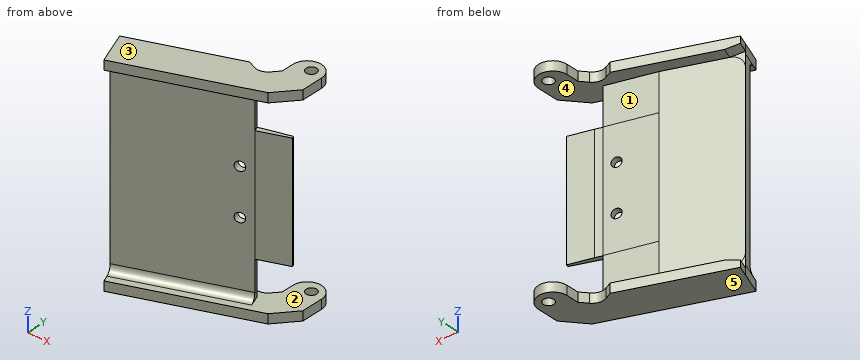
from build123d import *
from OCP.BRepFilletAPI import BRepFilletAPI_MakeChamfer

# Parameters (mm, degrees)
ESTRUSIONE_ESTRUSIONE1_DEPTH = 4
ESTRUSIONE_ESTRUSIONE2_DEPTH = 82
ESTRUSIONE_ESTRUSIONE3_START = 4
ESTRUSIONE_ESTRUSIONE3_DEPTH = 4
FORO_PER_VITE_M4_1_D         = 4.5
FORO_PER_VITE_M4_1_DEPTH     = 188
FORO_PER_VITE_M4_1_TIP       = 1.351936393
SCHIZZO6_W                   = 50
SCHIZZO6_H                   = 4
ESTRUSIONE_ESTRUSIONE4_DEPTH = 5
SMUSSO1_SIZE                 = 5.5
SMUSSO1_SIZE2                = 1.169061089
RACCORDO1_R                  = 3
SMUSSO2_SIZE                 = 5
RACCORDO2_START              = -86
RACCORDO2_DEPTH              = 4
RACCORDO2_2_DEPTH            = 4
SCHIZZO7_W                   = 50
SCHIZZO7_H                   = 2.5
ESTRUSIONE_ESTRUSIONE5_DEPTH = 13
SMUSSO3_SIZE                 = 20
SMUSSO3_SIZE_2               = 1.048155586
SMUSSO4_SIZE                 = 20
SMUSSO4_SIZE2                = 1.749773271
SMUSSO5_SIZE                 = 10
SMUSSO5_SIZE2                = 0.350328071
SCHIZZO8_R                   = 2
TAGLIO_ESTRUSIONE1_DEPTH     = 10


with BuildPart() as part:
    # Schizzo1 → Estrusione-Estrusione1 (new body)
    with BuildSketch(Plane.XY):
        with BuildLine():
            Line((4.891723927, 5.829729564), (4.891723927, 11.038087105))
            ThreePointArc((4.891723927, 11.038087105), (11.08058435, 17.226947528), (17.269444773, 11.038087105))
            Line((17.269444773, 11.038087105), (17.269444773, 1.912236928))
            Line((17.269444773, 1.912236928), (9.899185428, -6.871296125))
            Line((9.899185428, -6.871296125), (-42.94312967, -27.493410377))
            Line((-42.94312967, -27.493410377), (-46.57866514, -18.177677349))
            Line((-46.57866514, -18.177677349), (0, 0))
            Line((0, 0), (4.891723927, 5.829729564))
        make_face()
    extrude(amount=ESTRUSIONE_ESTRUSIONE1_DEPTH)

    # Schizzo4 → Estrusione-Estrusione2 (add)
    with BuildSketch(Plane.XY):
        Polygon((-45.124450952, -21.90397056), (1.454214188, -3.726293211), (0, 0), (-46.57866514, -18.177677349), align=None)
    extrude(amount=-ESTRUSIONE_ESTRUSIONE2_DEPTH)

    # Schizzo5 → Estrusione-Estrusione3 (add)
    with BuildSketch(Plane(origin=(0, 0, -82), x_dir=(-1, 0, 0), z_dir=(0, 0, -1)).offset(ESTRUSIONE_ESTRUSIONE3_START)):
        with BuildLine():
            Line((42.94312967, -27.493410377), (46.57866514, -18.177677349))
            Line((46.57866514, -18.177677349), (0, 0))
            Line((0, 0), (-4.891723927, 5.829729564))
            Line((-4.891723927, 5.829729564), (-4.891723927, 11.038087105))
            ThreePointArc((-4.891723927, 11.038087105), (-11.08058435, 17.226947528), (-17.269444773, 11.038087105))
            Line((-17.269444773, 11.038087105), (-17.269444773, 1.912236928))
            Line((-17.269444773, 1.912236928), (-9.899185428, -6.871296125))
            Line((-9.899185428, -6.871296125), (42.94312967, -27.493410377))
        make_face()
    extrude(amount=-ESTRUSIONE_ESTRUSIONE3_DEPTH)

    # Foro per Vite M4-1
    with Locations(Plane.XY.offset(4)):
        with Locations((11.891723927, 12.226947528)):
            Hole(FORO_PER_VITE_M4_1_D / 2, depth=FORO_PER_VITE_M4_1_DEPTH)
            with Locations((0, 0, -(FORO_PER_VITE_M4_1_DEPTH + FORO_PER_VITE_M4_1_TIP / 2))):  # 118° drill point
                Cone(0, FORO_PER_VITE_M4_1_D / 2, FORO_PER_VITE_M4_1_TIP, mode=Mode.SUBTRACT)

    # Schizzo6 → Estrusione-Estrusione4 (add)
    with BuildSketch(Plane(origin=(0, 0, 0), x_dir=(0.9315733027957475, 0.36355354697516373, 0), z_dir=(-0.36355354697516373, 0.9315733027957475, 0))):
        with Locations((-25, 84)):
            Rectangle(SCHIZZO6_W, SCHIZZO6_H)
        with Locations((-25, -2)):
            Rectangle(SCHIZZO6_W, SCHIZZO6_H)
    extrude(amount=ESTRUSIONE_ESTRUSIONE4_DEPTH)

    # Smusso1: one chamfer whose edges measure the first distance from different faces: ONE call of the kernel's chamfer builder (chamfer() names one face for all edges)
    smusso1_edges_1 = [part.edges().sort_by_distance(p)[0] for p in [
        (-47.487549007, -15.848744092, -82),
    ]]
    smusso1_side_1 = [part.faces().sort_by_distance(p)[0] for p in [
        (-24.198216437, -6.759905417, -82),
    ]]
    smusso1_edges_2 = [part.edges().sort_by_distance(p)[0] for p in [
        (-47.487549007, -15.848744092, 0),
    ]]
    smusso1_side_2 = [part.faces().sort_by_distance(p)[0] for p in [
        (-24.198216437, -6.759905417, 0),
    ]]
    smusso1 = BRepFilletAPI_MakeChamfer(part.part.solid().wrapped)
    for e in smusso1_edges_1:
        smusso1.Add(SMUSSO1_SIZE, SMUSSO1_SIZE2, e.wrapped, smusso1_side_1[0].wrapped)  # the first distance lies on this face
    for e in smusso1_edges_2:
        smusso1.Add(SMUSSO1_SIZE, SMUSSO1_SIZE2, e.wrapped, smusso1_side_2[0].wrapped)  # the first distance lies on this face
    add(Compound.cast(smusso1.Shape()), mode=Mode.REPLACE)

    # Raccordo1
    raccordo1_edges = [part.edges().sort_by_distance(p)[0] for p in [
        (-21.835118382, -12.815131886, -82),
        (-21.835118382, -12.815131886, 0),
    ]]
    fillet(raccordo1_edges, radius=RACCORDO1_R)

    # Smusso2
    smusso2_edges = [part.edges().sort_by_distance(p)[0] for p in [
        (-1.817767735, 4.657866514, 2),
        (-1.817767735, 4.657866514, -84),
    ]]
    chamfer(smusso2_edges, length=SMUSSO2_SIZE - 0.0001)  # a hair under: the kernel refuses the full size

    # Raccordo2: read off the stored shape, not the designer's step
    # Raccordo2 outline → Raccordo2 (add)
    with BuildSketch(Plane.XY.offset(RACCORDO2_START)):
        with BuildLine():
            Line((0, 0), (2.407895765, 2.869618428))
            ThreePointArc((2.407895765, 2.869618428), (-0.284030607, 1.214852073), (-3.430579557, 1.504591587))
            Line((-3.430579557, 1.504591587), (0, 0))
        make_face()
    extrude(amount=RACCORDO2_DEPTH)

    # Raccordo2 2 outline → Raccordo2 2 (add)
    with BuildSketch(Plane.XY):
        with BuildLine():
            Line((0, 0), (2.407895765, 2.869618428))
            ThreePointArc((2.407895765, 2.869618428), (-0.284030607, 1.214852073), (-3.430579557, 1.504591587))
            Line((-3.430579557, 1.504591587), (0, 0))
        make_face()
    extrude(amount=RACCORDO2_2_DEPTH)

    # Schizzo7 → Estrusione-Estrusione5 (add)
    with BuildSketch(Plane(origin=(0, 0, 0), x_dir=(0, 0, -1), z_dir=(0.9315733027957472, 0.3635535469751644, 0))):
        with Locations((41, -2.75)):
            Rectangle(SCHIZZO7_W, SCHIZZO7_H)
    extrude(amount=ESTRUSIONE_ESTRUSIONE5_DEPTH)

    # Smusso3
    # the kernel refuses this chamfer: 20, 1.048155586 mm, written as the material it takes off along each edge
    with BuildSketch(Plane(origin=(12.655783257, 3.328836156, -16), x_dir=(-0.9315733027957472, -0.3635535469751644, 0), z_dir=(0, 0, -1))) as smusso3_piece_1_section:
        Polygon((SMUSSO3_SIZE, 0), (0, -SMUSSO3_SIZE_2), (0, 0), align=None)
    smusso3_piece_1 = extrude(amount=50, mode=Mode.PRIVATE)
    smusso3_piece_1 = split(smusso3_piece_1, bisect_by=Plane(origin=(0.54533032, -1.397359954, -16), z_dir=(0.9315733027957472, 0.36355354697516445, 0)), keep=Keep.TOP, mode=Mode.PRIVATE)
    add(smusso3_piece_1, mode=Mode.SUBTRACT)

    # Smusso4
    smusso4_edges = [part.edges().sort_by_distance(p)[0] for p in [
        (0, 0, -41),
    ]]
    smusso4_side = [part.faces().sort_by_distance(p)[0] for p in [
        (-23.323124739, -9.102026325, -41),
    ]]
    chamfer(smusso4_edges, length=SMUSSO4_SIZE, length2=SMUSSO4_SIZE2, reference=smusso4_side[0])

    # Smusso5
    smusso5_edges = [part.edges().sort_by_distance(p)[0] for p in [
        (13.036843938, 2.352402395, -41),
    ]]
    smusso5_side = [part.faces().sort_by_distance(p)[0] for p in [
        (6.857772748, 0.306645312, -41),
    ]]
    chamfer(smusso5_edges, length=SMUSSO5_SIZE, length2=SMUSSO5_SIZE2, reference=smusso5_side[0])

    # Schizzo8 → Taglio-Estrusione1 (cut)
    with BuildSketch(Plane(origin=(0.489777192, -1.672892017, 0), x_dir=(0.9597141645441053, 0.2809781528400562, 0), z_dir=(-0.2809781528400562, 0.9597141645441053, 0))):
        with Locations(Location((-4.796849429, 31, 0), (0, 0, 180))):
            Circle(SCHIZZO8_R)
        with Locations(Location((-4.796849429, 51, 0), (0, 0, 180))):
            Circle(SCHIZZO8_R)
    extrude(amount=-TAGLIO_ESTRUSIONE1_DEPTH, mode=Mode.SUBTRACT)


solid = part.part
Model file for the job. Use its own axes, mm. Face numbers are marked on the shaded views. A direction names the side the tool comes from. Give positions to 0.01 mm unless a question says otherwise; leave off trailing zeros. Write each loop counter-clockwise with the first axis right and the second up, starting at its lowest first coordinate (ties: lowest second). Pieces come first, ordered by that corner, then holes. Notation, with made-up numbers: M 4.5,4.5 L 30.5,4.5 A36 ccw 30.5,43.5 Z; hole C 39,70.25 d4. An arc over 180 degrees is marked long. One line per item, written item: value. Start each with the question number.
Q1. Saw through at C-C, the plane y = 13.5. Write the cut outline in (x, z), plus the area to 3 significant figures.
Q2. Saw through at B-B, the plane x = 8. Write the cut outline in (y, z).
Q3. Two-plate mould, pull along Z, no slides. Class the marked faces 3, 4 and 5: +Z half, -Z half, draft (parallel to the pull), parting line (faces both ways), or undercut.
Q4. Saw through at A-A, the plane y = 8. Write the cut outline in (x, z), plus the area to 3 significant figures.
Q5. Saw through at D-D, the plane z = -67. Write the cut outline in (x, y), plus the area to 3 significant figures.
Q6. 3-axis set-ups, long thin cutter, end or side, ignore diameter. For the marked faces 1 and 2: which of +Z, -Z, +X, -X, +Y, -Y reach the whole face in a straight line?
Q7. Drop flat-ended pins along their axis: pin 1 Ø10 at (x, z) = (-23, -66) entering from -Y; pin 2 Ø6 at (x, y) = (11.89, 12.23) entering from +Z; pin 3 Ø1.5 at (y, z) = (2.5, -55) entering from +X; pin 4 Ø3 at (x, z) = (-9, -38.5) entering from -Y. Give the stop position or say it passes through.
Q8. Probe probe 1 along Z at (x, y) = (-15.5, -5.5); probe 2 along Y at (x, z) = (1.5, -24); probe 3 along Y at (x, z) = (-31, -58.5). List the from-to ranges inside material, lowest first. Write a range as [from, to].
Output values:
1. outline: M 5.4,-86 L 10.04,-86 L 10.04,-82 L 5.4,-82 Z; M 5.4,0 L 10.04,0 L 10.04,4 L 5.4,4 Z; M 13.75,-86 L 16.76,-86 L 16.76,-82 L 13.75,-82 Z; M 13.75,0 L 16.76,0 L 16.76,4 L 13.75,4 Z
1. area: 61.2 mm²
2. outline: M -7.61,-86 L 16.41,-86 L 16.41,-82 L -7.61,-82 Z; M -7.61,0 L 16.41,0 L 16.41,4 L -7.61,4 Z; M -1.17,-66 L 0.51,-66 L 0.51,-16 L -1.17,-16 Z
3. face 3: +Z half
3. face 4: undercut
3. face 5: -Z half
4. outline: M 4.89,-86 L 17.27,-86 L 17.27,-82 L 4.89,-82 Z; M 4.89,0 L 17.27,0 L 17.27,4 L 4.89,4 Z
4. area: 99.0 mm²
5. outline: M -46.58,-18.18 L -45.12,-21.9 L 1.45,-3.73 L 0.64,-1.63 L -18.63,-7.27 Z
5. area: 183 mm²
6. face 1: -X, +Y
6. face 2: none
7. pin 1: stops at y = -15.22
7. pin 2: stops at z = 4
7. pin 3: stops at x = 13.27
7. pin 4: stops at y = -8.39
8. probe 1: z = [-86, -82], [0, 4]
8. probe 2: y = [-3.71, -1.47]
8. probe 3: y = [-16.39, -12.1]
